from build123d import *

# Parameters (mm, degrees)
SKETCH1_R                    = 26.797
SKETCH1_R_2                  = 11.1125
BOSS_EXTRUDE1_DEPTH          = 11.938
SKETCH2_R                    = 12.827
CUT_EXTRUDE1_DEPTH           = 7.62
CHAMFER1_SIZE                = 0.762
SKETCH4_R                    = 3.3655
CUT_EXTRUDE2_DEPTH           = 12.938
CHAMFER2_SIZE                = 0.381
CIRPATTERN1_COUNT            = 4
CHAMFER2_OF_CIRPATTERN1_SIZE = 0.381
CUT_EXTRUDE5_DEPTH           = 0.79375


with BuildPart() as part:
    # Sketch1 → Boss-Extrude1 (new body)
    with BuildSketch(Plane(origin=(0, 0, 0), x_dir=(1, 0, 0), z_dir=(0, 1, 0))):
        Circle(SKETCH1_R)
        Circle(SKETCH1_R_2, mode=Mode.SUBTRACT)
    extrude(amount=BOSS_EXTRUDE1_DEPTH)

    # Sketch2 → Cut-Extrude1 (cut)
    with BuildSketch(Plane(origin=(0, 11.938, 0), x_dir=(1, 0, 0), z_dir=(0, 1, 0))):
        Circle(SKETCH2_R)
    extrude(amount=-CUT_EXTRUDE1_DEPTH, mode=Mode.SUBTRACT)

    # Chamfer1
    chamfer1_edges = [part.edges().sort_by_distance(p)[0] for p in [
        (-26.797, 0, 0),
        (-26.797, 11.938, 0),
    ]]
    chamfer(chamfer1_edges, length=CHAMFER1_SIZE)

    # Sketch3 → Cut-Revolve1 (revolve, cut)
    with BuildSketch(Plane.XY):
        Polygon((-16.51, 0), (-16.51, 1.2446), (-13.843, 0.6604), (-13.843, 1.27), (0, 1.27), (0, 0), align=None)
    revolve(axis=Axis((0, 11.938, 0), (0, -1, 0)), mode=Mode.SUBTRACT)

    # Sketch4 → Cut-Extrude2 (cut, through all)
    with BuildSketch(Plane(origin=(0, 0, 0), x_dir=(1, 0, 0), z_dir=(0, 1, 0))):
        with Locations((14.592916197, 14.592916197)):
            Circle(SKETCH4_R)
    cut_extrude2 = extrude(amount=CUT_EXTRUDE2_DEPTH, mode=Mode.SUBTRACT)

    # Chamfer2
    chamfer2_edges = [part.edges().sort_by_distance(p)[0] for p in [
        (11.227416197, 0, -14.592916197),
        (11.227416197, 11.938, -14.592916197),
    ]]
    chamfer(chamfer2_edges, length=CHAMFER2_SIZE)

    # CirPattern1: Cut-Extrude2 ×4 about axis
    cirpattern1_axis = Axis((0, 0, 0), (0, 1, 0))
    for i in range(1, CIRPATTERN1_COUNT):
        add(cut_extrude2.rotate(cirpattern1_axis, i * 360 / CIRPATTERN1_COUNT), mode=Mode.SUBTRACT)

    # Chamfer2 of CirPattern1
    chamfer2_of_cirpattern1_edges = [part.edges().sort_by_distance(p)[0] for p in [
        (-14.592916197, 0, -11.227416197),
        (-14.592916197, 11.938, -11.227416197),
        (-11.227416197, 0, 14.592916197),
        (-11.227416197, 11.938, 14.592916197),
        (14.592916197, 0, 11.227416197),
        (14.592916197, 11.938, 11.227416197),
    ]]
    chamfer(chamfer2_of_cirpattern1_edges, length=CHAMFER2_OF_CIRPATTERN1_SIZE)

    # Sketch5 → Cut-Extrude5 (cut, symmetric)
    with BuildSketch(Plane.XY):
        Polygon((-15.875, 0.931973496), (-28.575, 1.597552293), (-28.575, 0), (-15.875, 0), align=None)
    cut_extrude5 = extrude(amount=CUT_EXTRUDE5_DEPTH, both=True, mode=Mode.SUBTRACT)

    # Mirror1: Cut-Extrude5 across plane
    add(cut_extrude5.mirror(Plane(origin=(0, 0, 0), x_dir=(0, 0, 1), z_dir=(1, 0, 0))), mode=Mode.SUBTRACT)


solid = part.part
For this review, take the finished solid that the model builds, in its own axes (mm). A direction names the side the tool comes from. Coordinates: 2 decimals unless noted, no trailing zeros. Loops run counter-clockwise (first coordinate to the right, second up) from the corner with the lowest first, then second, coordinate; pieces in that order, holes last. Notation, with made-up numbers: (-1, 4) - (50, 4) arc R20 ccw to (50, 40) - close; hole circle Ø7 at (4.5, 8). An arc over 180 degrees is marked (long way). Use a Markdown table: item, result. Add a question column.
Item 1: For line 1 (Z direction, x = 0, y = 6.75); line 2 (X direction, y = 2.5, z = 11.5); line 3 (Z direction, x = -15.5, y = 3), list the stretches that pass through material, from the lowest coordinate up.
Item 2: We need section C-C (y = 8). Give the boundary of the cut face in (x, z), and give its area (3 significant figures).
Item 3: Tool access review of faces 1 (the face through (12.235, 8.181, -3.853)), 2 (the face through (-21.265, 5.896, 16.306)), 3 (the face through (21.57, 1.23, 0.01)): name each direction out of +Z, -Z, +X, -X, +Y, -Y from which nothing blocks a thin tool from reaching the whole face with its end or side.
Item 4: We need section A-A (x = 0). Give the boundary of the cut face in (y, z) (1 decimal), and give its area (3 significant figures).
Item 5: Insertion check: pin 1 Ø8 at (x, z) = (-4.5, -10.5) entering from +Y; pin 2 Ø14 at (x, z) = (3.5, -2.5) entering from -Y; pin 3 Ø1.5 at (x, y) = (-17.5, 3.5) entering from +Z; pin 4 Ø1 at (y, z) = (3, 13.5) entering from -X. Each pin has a flat end and moves straight along its axis. Give the tip position at first contact, or say it passes through.
Item 6: We need section D-D (z = -12). Give the number of separate pieces and of enclosed holes in the cut face, and give its area (3 significant figures).
Item 7: Mouldability with a two-part tool opening along X and no side actions: class faces 4 (the face through (-0.56, 0.12, 26.15)), 5 (the face through (-4, 4.318, -11)), 6 (the face through (22, 1, 0.794)) as pulls with the +X half, pulls with the -X half, needs draft (parallel to the pull), parting line crosses it, or undercut.
Results list:
| question | item | result |
|---|---|---|
| 1 | line 1 | z = -26.8 to -12.83, 12.83 to 26.8 |
| 1 | line 2 | x = -24.2 to -15.92, -13.27 to 13.27, 15.92 to 24.2 |
| 1 | line 3 | z = -21.86 to -17.83, -11.35 to 11.35, 17.83 to 21.86 |
| 2 | outline | circle Ø53.59 at (0, 0); hole circle Ø6.73 at (-14.59, -14.59); hole circle Ø6.73 at (-14.59, 14.59); hole circle Ø25.65 at (0, 0); hole circle Ø6.73 at (14.59, -14.59); hole circle Ø6.73 at (14.59, 14.59) |
| 2 | area | 1,600 mm^2 |
| 3 | face 1 | +Y |
| 3 | face 2 | +Y, -Y |
| 3 | face 3 | +X, -Y |
| 4 | outline | (0, -26) - (0.8, -26.8) - (11.2, -26.8) - (11.9, -26) - (11.9, -12.8) - (4.3, -12.8) - (4.3, -11.1) - (1.3, -11.1) - (1.3, -13.8) - (0.7, -13.8) - (1.2, -16.5) - (0, -16.5) - close; (0, 16.5) - (1.2, 16.5) - (0.7, 13.8) - (1.3, 13.8) - (1.3, 11.1) - (4.3, 11.1) - (4.3, 12.8) - (11.9, 12.8) - (11.9, 26) - (11.2, 26.8) - (0.8, 26.8) - (0, 26) - close |
| 4 | area | 335 mm^2 |
| 5 | pin 1 | stops at y = 11.94 |
| 5 | pin 2 | stops at y = 1.27 |
| 5 | pin 3 | stops at z = 20.92 |
| 5 | pin 4 | stops at x = -23.43 |
| 6 | separate pieces | 3 |
| 6 | enclosed holes | 0 |
| 6 | area | 373 mm^2 |
| 7 | face 4 | parting line crosses it |
| 7 | face 5 | undercut |
| 7 | face 6 | needs draft |
